Work out the finished part from the listing and answer in its coordinate system (mm). Face numbers are marked on the shaded views. A direction names the side the tool comes from. Coordinates: 2 decimals unless noted, no trailing zeros. Write each loop counter-clockwise with the first axis right and the second up, starting at its lowest first coordinate (ties: lowest second). Pieces come first, ordered by that corner, then holes. Notation, with made-up numbers: (44.5, 53) - (54.5, 53) arc R23 ccw to (54.5, 78) - close; hole circle Ø7 at (70, 5.25). An arc over 180 degrees is marked (long way). Use a Markdown table: item, result. Add a question column.
(1) The part is cut by section D-D, the plane y = 3.25. Give the vertices of the cut face in (x, z).
(2) The part is cut by section C-C, the plane x = 12.5. Give the vertices of the cut face in (y, z), then the cut area to 3 significant figures.
(3) Find the intervals of material crossed by line 1 (X direction, y = 2, z = 3.75); line 2 (X direction, y = 2.5, z = 2.25); line 3 (Y direction, x = 63, z = 7.25), in increasing order. Write a range as from..to.
(4) The part is cut by section B-B, the plane y = 8.75. Give the vertices of the cut face in (x, z).
(5) The part is cut by section A-A, the plane z = 5. Give the vertices of the cut face in (x, y), then the cut area to 3 significant figures.
(6) Given pin 1 Ø3 at (y, z) = (2.5, 4) entering from +X; pin 2 Ø3 at (x, z) = (30.1, 3.97) entering from +Y; pin 3 Ø4 at (y, z) = (8, 3) entering from -X; pin 4 Ø4 at (x, z) = (14.5, 5.5) entering from -Y, each flat-ended and moving along its own axis, determine where each tip first touches the part or whether it passes through.
(7) A tool of negligible diameter and unlimited length cuts with its end or side. For the marked faces 1, 2 and 3, from which of +Z, -Z, +X, -X, +Y, -Y can it reach the whole face along a straight path? Write none if from no direction.
Solid Edge part; units mm, degrees
sketch "Sketch1" plane through (0, 0, 0) normal (0, 0, 1) x (1, 0, 0)
  line L0 (0, 0) -> (0, 12.7)
  line L1 (0, 12.7) -> (79.248, 12.7)
  line L2 (79.248, 0) -> (79.248, 12.7)
  line L3 (79.248, 0) -> (0, 0)
  dimension "D1" = 79.248
extrude "Protrusion1" add sketch "Sketch1" along normal blind 7.9375
sketch "Sketch2" plane through (39.624, 6.35, 7.9375) normal (0, 0, 1) x (1, 0, 0)
  line L0 (-39.624, 1.27) -> (-15.875, 1.27)
  line L1 (-15.875, 1.27) -> (-15.875, -6.35)
  line L2 (-15.875, -6.35) -> (-39.624, -6.35)
  line L3 (-39.624, -6.35) -> (-39.624, 1.27)
  line L4 (15.875, -6.35) -> (15.875, 1.27)
  line L5 (15.875, 1.27) -> (39.624, 1.27)
  line L6 (39.624, 1.27) -> (39.624, -6.35)
  line L7 (39.624, -6.35) -> (15.875, -6.35)
  dimension "D1" = 15.875
  dimension "D2" = 39.624
extrude "Cutout1" cut sketch "Sketch2" against normal through all
hole "Hole_1" at (49.149, 0, 3.9687) direction (0, 1, 0) diameter 3.9675 end up to next
hole "Hole1" at (30.099, 0, 3.9688) direction (0, 1, 0) diameter 3.9675 end up to next
properties material "Aluminum, 6061-T6"
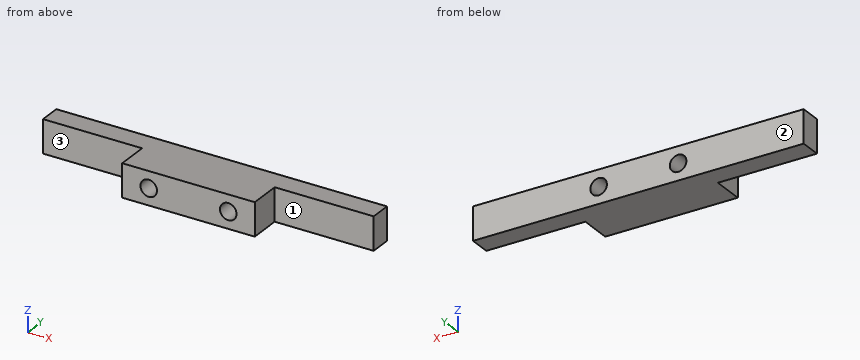
Model answer:
| question | item | result |
|---|---|---|
| 1 | outline | (23.75, 0) - (55.5, 0) - (55.5, 7.94) - (23.75, 7.94) - close; hole circle Ø3.97 at (30.1, 3.97); hole circle Ø3.97 at (49.15, 3.97) |
| 2 | outline | (7.62, 0) - (12.7, 0) - (12.7, 7.94) - (7.62, 7.94) - close |
| 2 | area | 40.3 mm^2 |
| 3 | line 1 | 23.75..28.13, 32.07..47.18, 51.12..55.5 |
| 3 | line 2 | 23.75..29.11, 31.09..48.16, 50.14..55.5 |
| 3 | line 3 | 7.62..12.7 |
| 4 | outline | (0, 0) - (79.25, 0) - (79.25, 7.94) - (0, 7.94) - close; hole circle Ø3.97 at (30.1, 3.97); hole circle Ø3.97 at (49.15, 3.97) |
| 5 | outline | (0, 7.62) - (23.75, 7.62) - (23.75, 0) - (28.4, 0) - (28.4, 12.7) - (0, 12.7) - close; (31.79, 0) - (47.45, 0) - (47.45, 12.7) - (31.79, 12.7) - close; (50.84, 0) - (55.5, 0) - (55.5, 7.62) - (79.25, 7.62) - (79.25, 12.7) - (50.84, 12.7) - close |
| 5 | area | 558 mm^2 |
| 6 | pin 1 | x = 55.5 |
| 6 | pin 2 | through |
| 6 | pin 3 | x = 0 |
| 6 | pin 4 | y = 7.62 |
| 7 | face 1 | +Z, -Z, +X, -Y |
| 7 | face 2 | +Z, -Z, +X, -X, +Y |
| 7 | face 3 | +Z, -Z, -X, -Y |
